Autodesk Inventor part; units mm, degrees
ref_plane "Work Plane1" through (0, 0, 2) normal (0, 0, 1) x (1, 0, 0)
ref_plane "YZ Plane" through (0, 0, 0) normal (1, 0, 0) x (0, 1, 0)
ref_plane "XZ Plane" through (0, 0, 0) normal (0, 1, 0) x (-1, 0, 0)
sketch "Sketch1" plane through (0, 0, 0) normal (0, 0, 1) x (1, 0, 0)
  circle A0 centre (0, 0) radius 30
  circle A1 centre (0, 0) radius 27
  circle A2 centre (0, 0) radius 5
  circle A3 centre (0, 0) radius 25
  dimension "d0" = 60
  dimension "d1" = 3
  dimension "d2" = 10
  dimension "d3" = 2
extrude "Extrusion1" add sketch "Sketch1" along normal blind 2 contours A0 | A1 | A3
extrude "Extrusion2" add sketch "Sketch1" along normal blind 4 contours A1
ref_plane "Work Plane1" through (0, 0, 2) normal (0, 0, 1) x (1, 0, 0)
sketch "Sketch2" plane through (0, 0, 2) normal (0, 0, 1) x (1, 0, 0)
  line L0 (-12.5, 32.3357) -> (12.5, 32.3357)
  line L1 (12.5, 32.3357) -> (12.5, 9.4484)
  line L2 (12.5, 9.4484) -> (-12.5, 9.4484)
  line L3 (-12.5, 9.4484) -> (-12.5, 32.3357)
  point P0 (0, 0)
  point P1 (0, 9.4484)
  dimension "d9" = 25
extrude "Extrusion3" cut sketch "Sketch2" along normal blind 4
properties part number "ServoHorn"
Part model, mm, in its own coordinate system. A direction names the side the tool comes from. Coordinates: 2 decimals unless noted, no trailing zeros. Order: outer loops, then holes, each group sorted by start corner. A loop starts at its lowest first (then second) coordinate and runs counter-clockwise, first axis right, second up. Notation, with made-up numbers: M -3.75,-35 L 5.25,-35 A35 ccw 5.25,4 Z; hole C 79.5,-25.75 d9. An arc over 180 degrees is marked long. Use a Markdown table: item, result.
(1) Cut at C-C on z = 0.6. Write the cut outline in (x, y).
A:
| item | result |
|---|---|
| outline | C 0,0 d60; hole C 0,0 d10 |
(2) Tool access for faces 1 (the cylindrical face through (1.01, -26.98, 2.99)), 2 (the flat face through (0, -6, 0)), 3 (the flat face through (-12.5, 23, 3)): list every direction of +Z, -Z, +X, -X, +Y, -Y with a clear straight run to the whole face (end or side of a thin tool).
A:
| item | result |
|---|---|
| face 1 | +Z |
| face 2 | -Z, +X, -X, +Y, -Y |
| face 3 | +Z, +Y |
(3) Probe L1, parallel to Y at x = 0, z = 0.45; L2, parallel to Z at x = -4.5, y = 7.5; L3, parallel to X at y = 22.5, z = 3.35. List the from-to ranges inside material, lowest first.
A:
| item | result |
|---|---|
| L1 | y = -30 to -5, 5 to 30 |
| L2 | z = 0 to 2 |
| L3 | x = -14.92 to -12.5, 12.5 to 14.92 |
(4) Flat gauge pins, fed straight in: pin 1 (1.6 mm diameter, centred on y = 23, z = 3, fed in from +X); pin 2 (1 mm diameter, centred on x = 21.5, y = 22, fed in from -Z); pin 3 (12 mm diameter, centred on x = 10.5, y = 12.5, fed in from +Z). Where does each tip first touch, or does it go through?
A:
| item | result |
|---|---|
| pin 1 | stops at x = 15.37 |
| pin 2 | passes through |
| pin 3 | stops at z = 2 |
(5) Cut at B-B on y = 0. Write the cut outline in (x, z), then the cut area to 3 significant figures.
A:
| item | result |
|---|---|
| outline | M -30,0 L -5,0 L -5,2 L -25,2 L -25,4 L -27,4 L -27,2 L -30,2 Z; M 5,0 L 30,0 L 30,2 L 27,2 L 27,4 L 25,4 L 25,2 L 5,2 Z |
| area | 108 mm^2 |
(6) Pull direction X, two halves, no side cores. Call faces 4 (the cylindrical face through (-29.97, -1.32, 0.99)), 5 (the flat face through (-8, -24, 4)), 6 (the flat face through (0, 7, 2)): released by +X, released by -X, zero draft, split by the parting line, or undercut.
A:
| item | result |
|---|---|
| face 4 | split by the parting line |
| face 5 | zero draft |
| face 6 | undercut |
(7) Cut at A-A on x = 0. Write the cut outline in (y, z).
A:
| item | result |
|---|---|
| outline | M -30,0 L -5,0 L -5,2 L -25,2 L -25,4 L -27,4 L -27,2 L -30,2 Z; M 5,0 L 30,0 L 30,2 L 5,2 Z |
(8) Cut at D-D on x = -8. Write the cut outline in (y, z).
A:
| item | result |
|---|---|
| outline | M -28.91,0 L 28.91,0 L 28.91,2 L -23.69,2 L -23.69,4 L -25.79,4 L -25.79,2 L -28.91,2 Z |
